CAD build for the part. Positions are in the model's coordinates, mm. A direction names the side the tool comes from. Round coordinates to 2 decimals unless told otherwise and drop trailing zeros. Loops run counter-clockwise (first coordinate to the right, second up) from the corner with the lowest first, then second, coordinate; pieces in that order, holes last.
```python
from build123d import *

# Parameters (mm, degrees)
SKETCH1_R           = 20.6248
BOSS_EXTRUDE1_DEPTH = 12.7
SKETCH2_R           = 8.73125
BOSS_EXTRUDE2_DEPTH = 203.2
SKETCH3_R           = 3.175
BOSS_EXTRUDE3_DEPTH = 25.4
SCALE1_SCALE        = 0.66


with BuildPart() as part:
    # Sketch1 → Boss-Extrude1 (new body)
    with BuildSketch(Plane.XY):
        Circle(SKETCH1_R)
    extrude(amount=-BOSS_EXTRUDE1_DEPTH)

    # Sketch2 → Boss-Extrude2 (add)
    with BuildSketch(Plane.XY):
        Circle(SKETCH2_R)
    extrude(amount=BOSS_EXTRUDE2_DEPTH)

    # Sketch3 → Boss-Extrude3 (add)
    with BuildSketch(Plane.XY.offset(203.2)):
        Circle(SKETCH3_R)
    extrude(amount=BOSS_EXTRUDE3_DEPTH)


with BuildPart() as part_1:
    # Scale1: scaled about (0, 0, 75.409153815)
    add(part.part.scale(SCALE1_SCALE).moved(Location((0, 0, 25.639112297))))


solid = part_1.part
```
Item 1: Cut at D-D, the plane y = -8. Give the cut face in (x, z).
Answers follow:
outline: (-11.01, 17.26) - (11.01, 17.26) - (11.01, 25.64) - (-11.01, 25.64) - close
Item 2: Cut at C-C, the plane z = 30.5. Give the cut face in (x, y), plus the area to 3 significant figures.
Answers follow:
outline: circle Ø11.53 at (0, 0)
area: 104 mm2
Item 3: Cut at A-A, the plane y = 0. Give the cut face in (x, z).
Answers follow:
outline: (-13.61, 17.26) - (13.61, 17.26) - (13.61, 25.64) - (5.76, 25.64) - (5.76, 159.75) - (2.1, 159.75) - (2.1, 176.52) - (-2.1, 176.52) - (-2.1, 159.75) - (-5.76, 159.75) - (-5.76, 25.64) - (-13.61, 25.64) - close
Item 4: Flat gauge pins, fed straight in: P1, Ø1, axis at x = 3.5, z = 103.5, coming from the -Y side; P2, Ø10, axis at x = -7.5, z = 110.5, coming from the +Y side; P3, Ø12, axis at y = 1, z = 115, coming from the +X side. Where does each tip first touch, or does it go through?
Answers follow:
P1: stops at y = -4.92
P2: stops at y = 5.19
P3: stops at x = 5.76
Item 5: 3-axis set-ups, long thin cutter, end or side, ignore diameter. For faces 1 (the flat face through (6, 0, 25.639)), 2 (the flat face through (0, 0, 17.257)): which of +Z, -Z, +X, -X, +Y, -Y reach the whole face in a straight line?
Answers follow:
face 1: +Z
face 2: -Z, +X, -X, +Y, -Y
Item 6: Probe line 1 (Z direction, x = -5.75, y = -10.5); line 2 (Z direction, x = 3.5, y = 3); line 3 (X direction, y = -0.5, z = 134). List the from-to ranges inside material, lowest first.
Answers follow:
line 1: z = 17.26 to 25.64
line 2: z = 17.26 to 159.75
line 3: x = -5.74 to 5.74
